Geometry: final body of the model. Coordinates: model frame, mm. A direction names the side the tool comes from. Round coordinates to 2 decimals unless told otherwise and drop trailing zeros. Loops run counter-clockwise (first coordinate to the right, second up) from the corner with the lowest first, then second, coordinate; pieces in that order, holes last. Notation, with made-up numbers: (22.25, -36) - (61.25, -36) arc R18 cw to (61.25, -11) - close; hole circle Ø8 at (77.5, 34). An arc over 180 degrees is marked (long way). Use CSV: the item, a comma, the result in double quotes.
from build123d import *

# Parameters (mm, degrees)
BOSS_EXTRUDE1_DEPTH = 10
BOSS_EXTRUDE2_START = 37
BOSS_EXTRUDE2_DEPTH = 3
LPATTERN1_COUNT     = 2
LPATTERN1_PITCH     = 11
SKETCH3_R           = 2.5
CUT_EXTRUDE1_DEPTH  = 40
SKETCH4_R           = 2.5
BOSS_EXTRUDE3_DEPTH = 3
LPATTERN2_COUNT     = 2
LPATTERN2_PITCH     = 37
SHELL2_START        = -8
SHELL2_DEPTH        = 16


# Read off the part's stored shape, not the designer's step: Shell2
with BuildPart() as part:
    # Sketch1 → Boss-Extrude1 (new, symmetric)
    with BuildSketch(Plane(origin=(0, 0, 0), x_dir=(1, 0, 0), z_dir=(0, 1, 0))):
        Polygon((0, 0), (0, 40), (40, 40), align=None)
    extrude(amount=BOSS_EXTRUDE1_DEPTH, both=True)

    # Sketch2 → Boss-Extrude2 (add)
    with BuildSketch(Plane(origin=(0, 0, 0), x_dir=(0, 0, -1), z_dir=(1, 0, 0)).offset(BOSS_EXTRUDE2_START)):
        with BuildLine():
            Line((40, 10), (50, 10))
            ThreePointArc((50, 10), (60, 0), (50, -10))
            Line((50, -10), (40, -10))
            Line((40, -10), (40, 10))
        make_face()
    boss_extrude2 = extrude(amount=-BOSS_EXTRUDE2_DEPTH)

    # LPattern1: Boss-Extrude2 ×2
    with Locations(*[(-i * LPATTERN1_PITCH, 0, 0) for i in range(1, LPATTERN1_COUNT)]):
        add(boss_extrude2)

    # Sketch3 → Cut-Extrude1 (cut)
    with BuildSketch(Plane(origin=(0, 0, 0), x_dir=(0, 0, -1), z_dir=(1, 0, 0))):
        with Locations((50, 0)):
            Circle(SKETCH3_R)
    extrude(amount=CUT_EXTRUDE1_DEPTH, mode=Mode.SUBTRACT)

    # Sketch4 → Boss-Extrude3 (add)
    with BuildSketch(Plane.XY):
        with BuildLine():
            Line((0, 10), (-10, 10))
            ThreePointArc((-10, 10), (-20, 0), (-10, -10))
            Line((-10, -10), (0, -10))
            Line((0, -10), (0, 10))
        make_face()
        with Locations((-10, 0)):
            Circle(SKETCH4_R, mode=Mode.SUBTRACT)
    boss_extrude3 = extrude(amount=-BOSS_EXTRUDE3_DEPTH)

    # LPattern2: Boss-Extrude3 ×2
    with Locations(*[(0, 0, -i * LPATTERN2_PITCH) for i in range(1, LPATTERN2_COUNT)]):
        add(boss_extrude3)

    # Shell2 outline → Shell2 (cut)
    with BuildSketch(Plane(origin=(0, 0, 0), x_dir=(1, 0, 0), z_dir=(0, 1, 0)).offset(SHELL2_START)):
        Polygon((35, 40), (25, 40), (25, 38), (0, 38), (0, 2.828427125), (35.171572875, 38), (35, 38), align=None)
    extrude(amount=SHELL2_DEPTH, mode=Mode.SUBTRACT)


solid = part.part
Item 1: Section B-B on x = -5.5. Return the cut outline in (y, z), plus the area to 3 significant figures.
Final values:
outline,"(-10, -40) - (10, -40) - (10, -37) - (-10, -37) - close; (-10, -3) - (10, -3) - (10, 0) - (-10, 0) - close"
area,"120 mm²"
Item 2: Section D-D on x = 7. Return the cut outline in (y, z), plus the area to 3 significant figures.
Final values:
outline,"(-10, -40) - (10, -40) - (10, -7) - (-10, -7) - close; hole (-8, -38) - (8, -38) - (8, -9.83) - (-8, -9.83) - close"
area,"209 mm²"
Item 3: Mould query, pull axis X, two halves, no side actions, for faces 1 (the cylindrical face through (-20, 0, -1)), 2 (the cylindrical face through (-12.5, 0.1, -38.5)), 3 (the flat face through (30, -9, -40)), 4 (the cylindrical face through (24.48, -0.96, -52.31)). Classes: released by +X, released by -X, zero draft, split by the parting line, or undercut.
Final values:
face 1,"released by -X"
face 2,"undercut"
face 3,"undercut"
face 4,"zero draft"
Item 4: Section C-C on y = 5.5. Return the cut outline in (x, z), plus the area to 3 significant figures.
Final values:
outline,"(-18.35, -40) - (23, -40) - (23, -58.35) - (26, -58.35) - (26, -40) - (25, -40) - (25, -38) - (0, -38) - (0, -37) - (-18.35, -37) - close; (-18.35, -3) - (0, -3) - (0, -2.83) - (35.17, -38) - (35, -38) - (35, -40) - (34, -40) - (34, -58.35) - (37, -58.35) - (37, -40) - (40, -40) - (0, 0) - (-18.35, 0) - close"
area,"382 mm²"
Item 5: Material intervals for line 1 (Y direction, x = 25, z = -50); line 2 (Y direction, x = 9, z = -16.5); line 3 (Z direction, x = -11, y = -8.75), sorted ascending.
Final values:
line 1,"y = -10 to -2.5, 2.5 to 10"
line 2,"y = -10 to -8, 8 to 10"
line 3,"z = -40 to -37, -3 to 0"
Item 6: Pin query (flat end, axial travel): P1, Ø2, axis at x = 25, y = 3.5, coming from the -Z side; P2, Ø1.5, axis at x = 28, y = -5, coming from the -Z side; P3, Ø0.6, axis at x = 29, y = -9, coming from the -Z side. Return the tip coordinate at first contact, or that it passes through.
Final values:
P1,"stops at z = -59.68"
P2,"stops at z = -31.58"
P3,"stops at z = -40"
Item 7: Section A-A on z = -46. Return the cut outline in (x, y).
Final values:
outline,"(23, -10) - (26, -10) - (26, 10) - (23, 10) - close; (34, -10) - (37, -10) - (37, 10) - (34, 10) - close"
Item 8: Reachability of faces 5 (the flat face through (35, 0, -39)), 6 (the flat face through (1, 0, -40)), 7 (the flat face through (38, 0, -40)) from +Z, -Z, +X, -X, +Y, -Y: full face, straight path, thin tool, end or side. Return the list, or none.
Final values:
face 5,"none"
face 6,"-Z, -X, +Y, -Y"
face 7,"-Z, +X, +Y, -Y"
